Source: CAD feature listing. Evaluate the final solid. Frame: model axes, mm. Face numbers are marked on the shaded views. A direction names the side the tool comes from. Round coordinates to 2 decimals unless told otherwise and drop trailing zeros. Loops run counter-clockwise (first coordinate to the right, second up) from the corner with the lowest first, then second, coordinate; pieces in that order, holes last. Notation, with made-up numbers: (89.25, -5.75) - (105.25, -5.75) arc R28 ccw to (105.25, 14.25) - close; hole circle Ø2 at (-9, 12.5). An arc over 180 degrees is marked (long way). One line per question, with ' | ' between items. Start each with the question number.
1. Cut plane C-C (x = 158.2). Return loops of the section in (y, z).
2. Cut plane D-D (z = 22.5). Return loops of the section in (x, y).
3. Pin query (flat end, axial travel): pin 1 (1.9 mm diameter, centred on y = 3.5, z = -59, fed in from -X); pin 2 (7 mm diameter, centred on x = 123.5, y = 3.5, fed in from -Z); pin 3 (10 mm diameter, centred on x = 156.5, z = 43, fed in from +Y); pin 4 (10 mm diameter, centred on x = 204, z = -35, fed in from -Y). Return the tip coordinate at first contact, or that it passes through.
4. Access query for the marked faces 1 and 2. Directions: +Z, -Z, +X, -X, +Y, -Y. A direction counts if a zero-diameter tool reaches every point of the face in a straight line with its end or side. Return the directions, or none.
5. Ray query, line 1 (Z direction, x = 268.6, y = 1.3); line 2 (Z direction, x = 268.6, y = 3.4); line 3 (X direction, y = 3.25, z = -73.7). Return the intervals inside material, ascending.
6. Cut plane A-A (z = 73.7). Return loops of the section in (x, y), then the cut area to 3 significant figures.
7. Cut plane B-B (z = -73.7). Return loops of the section in (x, y), then the cut area to 3 significant figures.
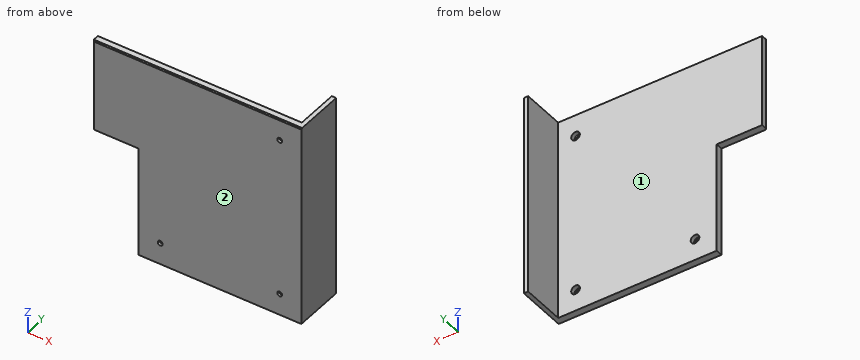
```python
from build123d import *

# Parameters (mm, degrees)
SKETCH1_W                      = 192.4
SKETCH1_H                      = 187.4
BOSS_EXTRUDE1_DEPTH            = 6.35
BOSS_EXTRUDE2_DEPTH            = 40
CUT_EXTRUDE1_REACH             = 142.122
SKETCH4_W                      = 42
SKETCH4_H                      = 102
CBORE_FOR_M4_SHCS1_D           = 4.5
CBORE_FOR_M4_SHCS1_CBORE_D     = 8
CBORE_FOR_M4_SHCS1_CBORE_DEPTH = 4
CHAMFER1_SIZE                  = 1


with BuildPart() as part:
    # Sketch1 → Boss-Extrude1 (new body)
    with BuildSketch(Plane(origin=(0, 0, 0), x_dir=(1, 0, 0), z_dir=(0, 1, 0))):
        Rectangle(SKETCH1_W, SKETCH1_H)
    extrude(amount=BOSS_EXTRUDE1_DEPTH)

    # Sketch2 → Boss-Extrude2 (add)
    with BuildSketch(Plane(origin=(0, 6.35, 0), x_dir=(1, 0, 0), z_dir=(0, 1, 0))):
        Polygon((-92.2, 89.7), (-92.2, -89.7), (-92.2, -93.7), (-96.2, -93.7), (-96.2, 93.7), (-92.2, 93.7), align=None)
    extrude(amount=BOSS_EXTRUDE2_DEPTH)

    # Sketch4 → Cut-Extrude1 (cut, up to next)
    with BuildSketch(Plane(origin=(0, 6.35, 0), x_dir=(1, 0, 0), z_dir=(0, 1, 0)), mode=Mode.PRIVATE) as cut_extrude1_sk1:
        with Locations((75.2, 42.7)):
            Rectangle(SKETCH4_W, SKETCH4_H)
    cut_extrude1_tool1 = extrude(cut_extrude1_sk1.sketch, amount=-CUT_EXTRUDE1_REACH, mode=Mode.PRIVATE) & part.part
    add(cut_extrude1_tool1.solids().sort_by_distance((75.2, 6.35, -42.7))[0], mode=Mode.SUBTRACT)

    # CBORE for M4 SHCS1 (through all)
    with Locations(Plane(origin=(0, 6.35, 0), x_dir=(1, 0, 0), z_dir=(0, 1, 0))):
        with Locations((34.2, 73.7), (-76.2, 73.7), (-76.2, -73.7)):
            CounterBoreHole(CBORE_FOR_M4_SHCS1_D / 2, CBORE_FOR_M4_SHCS1_CBORE_D / 2, CBORE_FOR_M4_SHCS1_CBORE_DEPTH)


with BuildPart() as body_2:
    # Mirror1: mirrored copy
    add(part.part.mirror(Plane(origin=(96.2, 6.35, -93.7), x_dir=(0, 0, 1), z_dir=(-1, 0, 0))))

    # Chamfer1
    chamfer1_edges = [body_2.edges().sort_by_distance(p)[0] for p in [
        (192.4, 0, 93.7),
        (96.2, 0, 51),
    ]]
    chamfer(chamfer1_edges, length=CHAMFER1_SIZE)


solid = body_2.part
```
Answers follow:
1) outline: (0, -93.7) - (6.35, -93.7) - (6.35, -77.7) - (2.35, -77.7) - (2.35, -75.95) - (0, -75.95) - close; (0, -71.45) - (2.35, -71.45) - (2.35, -69.7) - (6.35, -69.7) - (6.35, 93.7) - (1, 93.7) - (0, 92.7) - close
2) outline: (96.2, 1) - (97.2, 0) - (288.6, 0) - (288.6, 46.35) - (284.6, 46.35) - (284.6, 6.35) - (96.2, 6.35) - close
3) pin 1: stops at x = 138.2 | pin 2: stops at z = 8.3 | pin 3: stops at y = 6.35 | pin 4: stops at y = 0
4) face 1: +Z, -Z, -X, +Y | face 2: +Z, -Z, +X, -X, -Y
5) line 1: z = -93.7 to -75.95, -71.45 to 71.45, 75.95 to 93.7 | line 2: z = -93.7 to -77.7, -69.7 to 69.7, 77.7 to 93.7 | line 3: x = 138.2 to 154.2, 162.2 to 264.6, 272.6 to 288.6
6) outline: (96.2, 1) - (97.2, 0) - (266.35, 0) - (266.35, 2.35) - (264.6, 2.35) - (264.6, 6.35) - (96.2, 6.35) - close; (270.85, 0) - (288.6, 0) - (288.6, 46.35) - (284.6, 46.35) - (284.6, 6.35) - (272.6, 6.35) - (272.6, 2.35) - (270.85, 2.35) - close | area: 1,340 mm2
7) outline: (138.2, 0) - (155.95, 0) - (155.95, 2.35) - (154.2, 2.35) - (154.2, 6.35) - (138.2, 6.35) - close; (160.45, 0) - (266.35, 0) - (266.35, 2.35) - (264.6, 2.35) - (264.6, 6.35) - (162.2, 6.35) - (162.2, 2.35) - (160.45, 2.35) - close; (270.85, 0) - (288.6, 0) - (288.6, 46.35) - (284.6, 46.35) - (284.6, 6.35) - (272.6, 6.35) - (272.6, 2.35) - (270.85, 2.35) - close | area: 1,030 mm2
